```python
from build123d import *

# Parameters (mm, degrees)
BOSS_EXTRUDE1_DEPTH      = 18
BOSS_EXTRUDE2_DEPTH      = 2
BOSS_EXTRUDE2_DEPTH_BACK = 2
SKETCH2_W                = 8
SKETCH2_H                = 10
SKETCH2_R                = 2.3


with BuildPart() as part:
    # Sketch1 → Boss-Extrude1 (new body)
    with BuildSketch(Plane.XY):
        Polygon((0, 0), (0, 18), (12, 0), align=None)
    extrude(amount=BOSS_EXTRUDE1_DEPTH)

    # Sketch2 → Boss-Extrude2 (add, two sides: drawn at the far end of the back side and taken through both)
    with BuildSketch(Plane.XY.offset(9).offset(-BOSS_EXTRUDE2_DEPTH_BACK)):
        with Locations((6, -5)):
            Rectangle(SKETCH2_W, SKETCH2_H)
        with Locations((6, -5)):
            Circle(SKETCH2_R, mode=Mode.SUBTRACT)
    extrude(amount=BOSS_EXTRUDE2_DEPTH + BOSS_EXTRUDE2_DEPTH_BACK)


solid = part.part
```
Input: part model. Units: mm. Frame: model coordinates. A direction names the side the tool comes from. Coordinates: 2 decimals unless noted, no trailing zeros. Loops run counter-clockwise (first coordinate to the right, second up) from the corner with the lowest first, then second, coordinate; pieces in that order, holes last. Notation, with made-up numbers: (7, 20.25) - (35, 20.25) arc R24 ccw to (35, 50.25) - close; hole circle Ø11 at (14, 28). An arc over 180 degrees is marked (long way). Answer in a Markdown table with one row per item.
(1) Material intervals for L1, parallel to Y at x = 6, z = 9.45; L2, parallel to X at y = -7, z = 10; L3, parallel to Y at x = 7.25, z = 15.75 (3 decimals), sorted ascending. Write a range as from..to.
Model answer:
| item | result |
|---|---|
| L1 | y = -10..-7.3, -2.7..9 |
| L2 | x = 2..4.86, 7.14..10 |
| L3 | y = 0..7.125 |
(2) Cut plane B-B on x = 6. Output: boundary loops of the cut face in (y, z), plus the area to 3 significant figures.
Model answer:
| item | result |
|---|---|
| outline | (-10, 7) - (-7.3, 7) - (-7.3, 11) - (-10, 11) - close; (-2.7, 7) - (0, 7) - (0, 0) - (9, 0) - (9, 18) - (0, 18) - (0, 11) - (-2.7, 11) - close |
| area | 184 mm² |
(3) Cut plane D-D on z = 13.5. Output: boundary loops of the cut face in (x, y), plus the area to 3 significant figures.
Model answer:
| item | result |
|---|---|
| outline | (0, 0) - (12, 0) - (0, 18) - close |
| area | 108 mm² |
(4) Mould query, pull axis Y, two halves, no side actions, for faces 1 (the face through (6, -10, 9)), 2 (the face through (7.06, -7.04, 8.97)), 3 (the face through (5.1, -2.7, 7)). Classes: pulls with the +Y half, pulls with the -Y half, needs draft (parallel to the pull), parting line crosses it, or undercut.
Model answer:
| item | result |
|---|---|
| face 1 | pulls with the -Y half |
| face 2 | undercut |
| face 3 | needs draft |
(5) Set-up query: faces 4 (the face through (2, -5, 9)), 5 (the face through (0, 9, 9)), 6 (the face through (5.1, -2.7, 11)), 7 (the face through (10, -5, 9)). Return all of +Z, -Z, +X, -X, +Y, -Y with unobstructed straight access to the full face (end or side cutting, diameter ignored); none if empty.
Model answer:
| item | result |
|---|---|
| face 4 | +Z, -Z, -X, -Y |
| face 5 | +Z, -Z, -X, +Y, -Y |
| face 6 | +Z, +X, -X, -Y |
| face 7 | +Z, -Z, +X, -Y |
(6) Cut plane C-C on x = 2.5. Output: boundary loops of the cut face in (y, z).
Model answer:
| item | result |
|---|---|
| outline | (-10, 7) - (0, 7) - (0, 0) - (14.25, 0) - (14.25, 18) - (0, 18) - (0, 11) - (-10, 11) - close |
(7) Pin query (flat end, axial travel): P1, Ø4.5, axis at y = -6, z = 9.5, coming from the +X side; P2, Ø8, axis at y = 5.5, z = 5.5, coming from the +X side; P3, Ø3, axis at y = -6, z = 8, coming from the -X side; P4, Ø3, axis at x = 6, y = -5, coming from the +Z side. Return the tip coordinate at first contact, or that it passes through.
Model answer:
| item | result |
|---|---|
| P1 | stops at x = 10 |
| P2 | stops at x = 11 |
| P3 | stops at x = 2 |
| P4 | passes through |
(8) Cut plane A-A on y = -5. Output: boundary loops of the cut face in (x, z), plus the area to 3 significant figures.
Model answer:
| item | result |
|---|---|
| outline | (2, 7) - (3.7, 7) - (3.7, 11) - (2, 11) - close; (8.3, 7) - (10, 7) - (10, 11) - (8.3, 11) - close |
| area | 13.6 mm² |
